Input: part model. Units: mm. Frame: model coordinates. A direction names the side the tool comes from. Coordinates: 2 decimals unless noted, no trailing zeros. Order: outer loops, then holes, each group sorted by start corner. A loop starts at its lowest first (then second) coordinate and runs counter-clockwise, first axis right, second up.
from build123d import *

# Parameters (mm, degrees)
SKETCH1_R           = 47.5
BOSS_EXTRUDE1_DEPTH = 440
SKETCH2_R           = 30
BOSS_EXTRUDE2_DEPTH = 50
SKETCH3_R           = 30
BOSS_EXTRUDE3_DEPTH = 50
SKETCH4_R           = 25
BOSS_EXTRUDE4_DEPTH = 10
SKETCH5_R           = 25
BOSS_EXTRUDE5_DEPTH = 10


with BuildPart() as part:
    # Sketch1 → Boss-Extrude1 (new body)
    with BuildSketch(Plane.XY):
        Circle(SKETCH1_R)
    extrude(amount=BOSS_EXTRUDE1_DEPTH)

    # Sketch2 → Boss-Extrude2 (add)
    with BuildSketch(Plane(origin=(0, 0, 0), x_dir=(-1, 0, 0), z_dir=(0, 0, -1))):
        Circle(SKETCH2_R)
    extrude(amount=BOSS_EXTRUDE2_DEPTH)

    # Sketch3 → Boss-Extrude3 (add)
    with BuildSketch(Plane.XY.offset(440)):
        Circle(SKETCH3_R)
    extrude(amount=BOSS_EXTRUDE3_DEPTH)

    # Sketch4 → Boss-Extrude4 (add)
    with BuildSketch(Plane.XY.offset(490)):
        Circle(SKETCH4_R)
    extrude(amount=BOSS_EXTRUDE4_DEPTH)

    # Sketch5 → Boss-Extrude5 (add)
    with BuildSketch(Plane(origin=(0, 0, -50), x_dir=(-1, 0, 0), z_dir=(0, 0, -1))):
        Circle(SKETCH5_R)
    extrude(amount=BOSS_EXTRUDE5_DEPTH)


solid = part.part
Item 1: Ray query, probe 1 along Z at (x, y) = (40.5, 21); probe 2 along X at (y, z) = (-2.5, 116.5); probe 3 along X at (y, z) = (0.5, 224.5). Return the intervals inside material, ascending.
Response values:
probe 1: z = 0 to 440
probe 2: x = -47.43 to 47.43
probe 3: x = -47.5 to 47.5
Item 2: Access query for faces 1 (the face through (23.846, 7.509, 494.93)), 2 (the face through (0, 0, -60)), 3 (the face through (7, 25, -50)). Directions: +Z, -Z, +X, -X, +Y, -Y. A direction counts if a zero-diameter tool reaches every point of the face in a straight line with its end or side. Return the directions, or none.
Response values:
face 1: +Z
face 2: -Z, +X, -X, +Y, -Y
face 3: -Z
Item 3: Cut plane A-A on x = 0. Return loops of the section in (y, z).
Response values:
outline: (-47.5, 0) - (-30, 0) - (-30, -50) - (-25, -50) - (-25, -60) - (25, -60) - (25, -50) - (30, -50) - (30, 0) - (47.5, 0) - (47.5, 440) - (30, 440) - (30, 490) - (25, 490) - (25, 500) - (-25, 500) - (-25, 490) - (-30, 490) - (-30, 440) - (-47.5, 440) - close
Item 4: Pin query (flat end, axial travel): pin 1 Ø1 at (x, y) = (-12, 30) entering from +Z; pin 2 Ø8 at (x, z) = (35.5, 213.5) entering from +Y; pin 3 Ø1.5 at (y, z) = (-8.5, 28.5) entering from +X. Return the tip coordinate at first contact, or that it passes through.
Response values:
pin 1: stops at z = 440
pin 2: stops at y = 35.55
pin 3: stops at x = 46.86
Item 5: Cut plane C-C on z = 165.5. Return loops of the section in (x, y), then the cut area to 3 significant figures.
Response values:
outline: circle Ø95 at (0, 0)
area: 7,090 mm2
Item 6: Cut plane D-D on z = 453.5. Return loops of the section in (x, y).
Response values:
outline: circle Ø60 at (0, 0)
